```python
from build123d import *

# Parameters (mm, degrees)
BOSS_EXTRUDE2_DEPTH = 2.6
SKETCH15_OUTSIDE_W  = 18.79
SKETCH15_OUTSIDE_H  = 17.568
SKETCH15_OUTSIDE_R  = 3.95
CUT_EXTRUDE4_DEPTH  = 2.6
CUT_EXTRUDE4_DRAFT  = -45
SKETCH16_OUTSIDE_W  = 18.79
SKETCH16_OUTSIDE_H  = 17.568
SKETCH16_OUTSIDE_R  = 3.95
CUT_EXTRUDE5_DEPTH  = 2.6
CUT_EXTRUDE5_DRAFT  = -45


with BuildPart() as part:
    # Sketch2 → Boss-Extrude2 (new body)
    with BuildSketch(Plane(origin=(0, 0, 0), x_dir=(1, 0, 0), z_dir=(0, 1, 0))):
        Polygon((-4.561067127, 0), (-2.280533563, -3.95), (2.280533563, -3.95), (4.561067127, 0), (2.280533563, 3.95), (-2.280533563, 3.95), align=None)
    extrude(amount=BOSS_EXTRUDE2_DEPTH)

    # Sketch13 → Cut-Revolve1 (revolve, cut)
    with BuildSketch(Plane.XY, mode=Mode.PRIVATE) as cut_revolve1_sk:
        Polygon((0, 2.6), (2.217, 2.6), (2.150316044, 2.5615), (2.150316044, 2.5385), (2.563410162, 2.3), (2.150316044, 2.0615), (2.150316044, 2.0385), (2.563410162, 1.8), (2.150316044, 1.5615), (2.150316044, 1.5385), (2.563410162, 1.3), (2.150316044, 1.0615), (2.150316044, 1.0385), (2.563410162, 0.8), (2.150316044, 0.5615), (2.150316044, 0.5385), (2.563410162, 0.3), (2.150316044, 0.0615), (2.150316044, 0.0385), (2.217, 0), (0, 0), align=None)
    revolve(cut_revolve1_sk.sketch.rotate(Axis((0, 4.352000656, 0), (0, -1, 0)), 180), axis=Axis((0, 4.352000656, 0), (0, -1, 0)), mode=Mode.SUBTRACT)


with BuildPart() as cut_extrude4_tool:
    # Sketch15 outside → Cut-Extrude4 (with draft: the straight prism first)
    with BuildSketch(Plane(origin=(0, 2.6, 0), x_dir=(1, 0, 0), z_dir=(0, 1, 0))):
        Rectangle(SKETCH15_OUTSIDE_W, SKETCH15_OUTSIDE_H)
        Circle(SKETCH15_OUTSIDE_R, mode=Mode.SUBTRACT)
    extrude(amount=-CUT_EXTRUDE4_DEPTH)
    # Cut-Extrude4: the draft: its side faces are tilted about the plane it starts from
    cut_extrude4_sides = [cut_extrude4_tool.faces().sort_by_distance(p)[0] for p in [
        (0, 1.3, 8.784),
        (9.395, 1.3, 0),
        (0, 1.3, -8.784),
        (-9.395, 1.3, 0),
        (-3.95, 1.3, 0),
    ]]
    draft(cut_extrude4_sides, Plane(origin=(0, 2.6, 0), x_dir=(1, 0, 0), z_dir=(0, 1, 0)), CUT_EXTRUDE4_DRAFT)


with BuildPart() as part_1:
    add(part.part)

    # Cut-Extrude4: cut by cut_extrude4_tool
    add(cut_extrude4_tool.part, mode=Mode.SUBTRACT)


with BuildPart() as cut_extrude5_tool:
    # Sketch16 outside → Cut-Extrude5 (with draft: the straight prism first)
    with BuildSketch(Plane.XZ):
        Rectangle(SKETCH16_OUTSIDE_W, SKETCH16_OUTSIDE_H)
        Circle(SKETCH16_OUTSIDE_R, mode=Mode.SUBTRACT)
    extrude(amount=-CUT_EXTRUDE5_DEPTH)
    # Cut-Extrude5: the draft: its side faces are tilted about the plane it starts from
    cut_extrude5_sides = [cut_extrude5_tool.faces().sort_by_distance(p)[0] for p in [
        (0, 1.3, -8.784),
        (9.395, 1.3, 0),
        (0, 1.3, 8.784),
        (-9.395, 1.3, 0),
        (-3.95, 1.3, 0),
    ]]
    draft(cut_extrude5_sides, Plane.XZ, CUT_EXTRUDE5_DRAFT)


with BuildPart() as part_2:
    add(part_1.part)

    # Cut-Extrude5: cut by cut_extrude5_tool
    add(cut_extrude5_tool.part, mode=Mode.SUBTRACT)


solid = part_2.part
```
Geometry check sheet. Reference: the model listing, model coordinates, mm. Coordinates: 2 decimals unless noted, no trailing zeros. Order: outer loops, then holes, each group sorted by start corner. A loop starts at its lowest first (then second) coordinate and runs counter-clockwise, first axis right, second up. Notation, with made-up numbers: (38, 52.25) - (91, 52.25) arc R29 ccw to (91, 84.25) - close; hole circle Ø5 at (78, 11.5). An arc over 180 degrees is marked (long way). Answer in a Markdown table with one row per item. Add a question column.
1. Section check A-A (y = 1.4). Enter the section's corners in (x, z).
2. Material ranges on L1, parallel to Z at x = 0, y = 0.6; L2, parallel to Y at x = 1.25, z = 2; L3, parallel to Z at x = 1.5, y = 0.75, recorded low to high. Write a range as [from, to].
3. Gauge pin test, flat end, axial feed: pin 1 Ø3.5 at (x, z) = (0, 0) entering from +Y. Record the tip position at first contact, or that the pin passes through.
4. Section check B-B (y = 2.4). Enter the section's corners in (x, z), plus the area to 3 significant figures.
Data:
| question | item | result |
|---|---|---|
| 1 | outline | (-4.56, 0) - (-2.28, -3.95) - (2.28, -3.95) - (4.56, 0) - (2.28, 3.95) - (-2.28, 3.95) - close; hole circle Ø4.78 at (0, 0) |
| 2 | L1 | z = [-3.95, -2.22], [2.22, 3.95] |
| 2 | L2 | y = [0, 0.18], [0.42, 0.68], [0.92, 1.18], [1.42, 1.68], [1.92, 2.18], [2.42, 2.6] |
| 2 | L3 | z = [-3.95, -1.97], [1.97, 3.95] |
| 3 | pin 1 | passes through |
| 4 | outline | (-4.06, -0.87) - (-2.78, -3.08) arc R4.15 ccw to (-1.27, -3.95) - (1.27, -3.95) arc R4.15 ccw to (2.78, -3.08) - (4.06, -0.87) arc R4.15 ccw to (4.06, 0.87) - (2.78, 3.08) arc R4.15 ccw to (1.27, 3.95) - (-1.27, 3.95) arc R4.15 ccw to (-2.78, 3.08) - (-4.06, 0.87) arc R4.15 ccw to start; hole circle Ø4.78 at (0, 0) |
| 4 | area | 34.1 mm² |
